Geometry check sheet. Reference: the model listing, model coordinates, mm. Round coordinates to 2 decimals unless told otherwise and drop trailing zeros. Write each loop counter-clockwise with the first axis right and the second up, starting at its lowest first coordinate (ties: lowest second). Pieces come first, ordered by that corner, then holes.
from build123d import *

# Parameters (mm, degrees)
F1_DEPTH = 10
F2_R     = 5
F2_R_2   = 5.0000678119
F3_DEPTH = 25


with BuildPart() as f1:
    # F0 (on Top) → F1 (new body)
    with BuildSketch(Plane.XY):
        Polygon((10, 127.279220223), (-10, 127.279220223), (53.6396103068, 63.6396103068), (63.6396102761, 73.6396102761), align=None)
        Polygon((63.6396102761, 73.6396102761), (53.6396103068, 63.6396103068), (63.6396103375, 53.6396103375), (73.6396103068, 63.6396103068), align=None)
        Polygon((117.2792206136, 127.2792206136), (63.6396102761, 73.6396102761), (73.6396103068, 63.6396103068), (137.2792206136, 127.2792206136), align=None)
        Polygon((73.6396103068, 63.6396103068), (63.6396103375, 53.6396103375), (117.2792210042, 0), (137.2792210042, 0), align=None)
        Polygon((63.6396103375, 53.6396103375), (53.6396103068, 63.6396103068), (-10, 0), (10, 0), align=None)
    extrude(amount=F1_DEPTH)

    # F2 (on face) → F3 (cut)
    with BuildSketch(Plane.XY.offset(10)):
        with Locations((7.0710959132, 120.208220223)):
            Circle(F2_R)
        with Locations((120.2081528017, 120.2081528017)):
            Circle(F2_R_2)
        with Locations((120.2083168306, 7.071)):
            Circle(F2_R)
        with Locations((7.0710959005, 7.071)):
            Circle(F2_R)
    extrude(amount=-F3_DEPTH, mode=Mode.SUBTRACT)


solid = f1.part
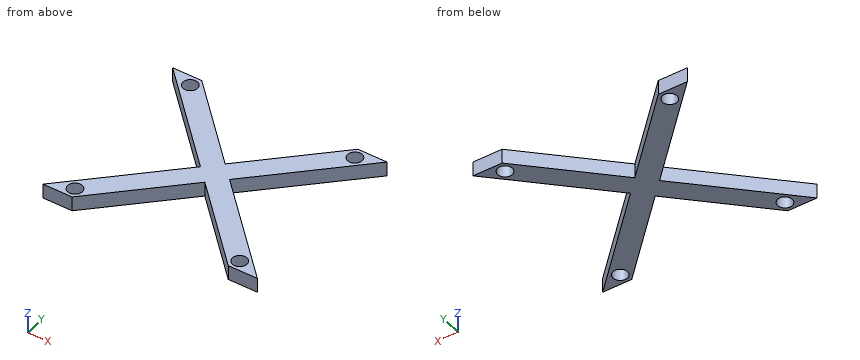
1. Section check D-D (z = 5.5). Record the cut outline in (x, y), plus the area to 3 significant figures.
2. Section check C-C (y = 25). Record the cut outline in (x, z).
3. Section check A-A (x = 6). Record the cut outline in (y, z), plus the area to 3 significant figures.
4. Depth check by flat-ended pin: pin 1 Ø4 at (x, z) = (113, 5.5) entering from -Y; pin 2 Ø6 at (x, y) = (7.07, 7.07) entering from -Z; pin 3 Ø5 at (x, z) = (19.5, 2.5) entering from +Y; pin 4 Ø1.5 at (y, z) = (59.5, 7.5) entering from +X. Enter the tip coordinate at first touch or a pass-through.
5. Section check B-B (x = 31). Record the cut outline in (y, z).
6. Scan lines: line 1 along Y through (x, z) = (10, 6.25); line 2 along X through (y, z) = (15, 7.5); line 3 along Y through (x, z) = (6, 6.75). Record each from-to range of solid material in increasing order.
Results below:
1. outline: (-10, 0) - (10, 0) - (63.64, 53.64) - (117.28, 0) - (137.28, 0) - (73.64, 63.64) - (137.28, 127.28) - (117.28, 127.28) - (63.64, 73.64) - (10, 127.28) - (-10, 127.28) - (53.64, 63.64) - close; hole circle Ø10 at (7.07, 7.07); hole circle Ø10 at (7.07, 120.21); hole circle Ø10 at (120.21, 7.07); hole circle Ø10 at (120.21, 120.21)
1. area: 4,580 mm2
2. outline: (15, 0) - (35, 0) - (35, 10) - (15, 10) - close; (92.28, 0) - (112.28, 0) - (112.28, 10) - (92.28, 10) - close
3. outline: (0, 0) - (2.19, 0) - (2.19, 10) - (0, 10) - close; (11.95, 0) - (16, 0) - (16, 10) - (11.95, 10) - close; (111.28, 0) - (115.32, 0) - (115.32, 10) - (111.28, 10) - close; (125.09, 0) - (127.28, 0) - (127.28, 10) - (125.09, 10) - close
3. area: 125 mm2
4. pin 1: stops at y = 2.28
4. pin 2: passes through
4. pin 3: stops at y = 120.28
4. pin 4: stops at x = 78.53
5. outline: (21, 0) - (41, 0) - (41, 10) - (21, 10) - close; (86.28, 0) - (106.28, 0) - (106.28, 10) - (86.28, 10) - close
6. line 1: y = 0 to 3.02, 11.12 to 20, 107.28 to 116.16, 124.26 to 127.28
6. line 2: x = 5 to 25, 102.28 to 122.28
6. line 3: y = 0 to 2.19, 11.95 to 16, 111.28 to 115.32, 125.09 to 127.28
